```python
from build123d import *

# Parameters (mm, degrees)
SKETCH1_W           = 80
SKETCH1_H           = 40
BOSS_EXTRUDE1_DEPTH = 3
SKETCH2_W           = 80
SKETCH2_H           = 3
BOSS_EXTRUDE2_DEPTH = 12
SKETCH3_R           = 2
CUT_EXTRUDE1_DEPTH  = 12


with BuildPart() as part:
    # Sketch1 → Boss-Extrude1 (new body)
    with BuildSketch(Plane.XY):
        Rectangle(SKETCH1_W, SKETCH1_H)
    extrude(amount=BOSS_EXTRUDE1_DEPTH)

    # Sketch2 → Boss-Extrude2 (add)
    with BuildSketch(Plane.XY.offset(3)):
        with Locations((0, 18.5)):
            Rectangle(SKETCH2_W, SKETCH2_H)
    extrude(amount=BOSS_EXTRUDE2_DEPTH)

    # Sketch3 → Cut-Extrude1 (cut)
    with BuildSketch(Plane(origin=(0, 20, 0), x_dir=(1, 0, 0), z_dir=(0, 1, 0))):
        with Locations(Location((15, -8.5, 0), (0, 0, 270))):
            Circle(SKETCH3_R)
        with Locations(Location((-20, -8.5, 0), (0, 0, 270))):
            Circle(SKETCH3_R)
    extrude(amount=-CUT_EXTRUDE1_DEPTH, mode=Mode.SUBTRACT)


solid = part.part
```
Could you check a few things on this model? Use its own coordinates, in mm. A direction names the side the tool comes from. Give positions to 0.01 mm unless a question says otherwise; leave off trailing zeros. Loops run counter-clockwise (first coordinate to the right, second up) from the corner with the lowest first, then second, coordinate; pieces in that order, holes last. Notation, with made-up numbers: (86, 88) - (96, 88) arc R14 ccw to (96, 110) - close; hole circle Ø9 at (0, 88.5). An arc over 180 degrees is marked (long way). Answer in a Markdown table with one row per item. Add a question column.
Q1. For pin 1 (8 mm diameter, centred on y = -4, z = 4, fed in from -X); pin 2 (3 mm diameter, centred on x = -6, z = 9.5, fed in from -Y); pin 3 (3 mm diameter, centred on x = -20, z = 8.5, fed in from +Y); pin 4 (11 mm diameter, centred on x = 2.5, y = 7, fed in from +Z), each with a flat end and sliding along its axis, tell me the tip position at first contact or that it passes through.
Q2. Please list where these lines run through material, in increasing order: L1, parallel to X at y = 19.2, z = 8.5; L2, parallel to Y at x = -24.5, z = 13.5; L3, parallel to Z at x = 12, y = -10. Write a range as from..to.
Q3. If we section it at B-B (z = 8.5): List the corners of the cut face in (x, y) for me, plus the area to 3 significant figures.
Q4. If we section it at C-C (x = -2): List the corners of the cut face in (y, z) for me, plus the area to 3 significant figures.
Q5. If we section it at A-A (x = -20): List the corners of the cut face in (y, z) for me.
Q6. We'd pull the mould along Z, two halves only. Please class faces 1 (the face through (-1, -1, 3)), 2 (the face through (-18.017, 18.521, 8.24)), 3 (the face through (-40, 4, 2)): +Z half, -Z half, draft (parallel to the pull), parting line (faces both ways), or undercut.
Q7. If we section it at D-D (y = -2.5): List the corners of the cut face in (x, z) for me.
Q8. Which directions (+Z, -Z, +X, -X, +Y, -Y) give clear straight access to the entire face, cutting with the end or side of a thin tool? Please do faces 4 (the face through (-1, 17, 9)), 5 (the face through (-1, 0, 0)).
The answers:
| question | item | result |
|---|---|---|
| 1 | pin 1 | stops at x = -40 |
| 1 | pin 2 | stops at y = 17 |
| 1 | pin 3 | passes through |
| 1 | pin 4 | stops at z = 3 |
| 2 | L1 | x = -40..-22, -18..13, 17..40 |
| 2 | L2 | y = 17..20 |
| 2 | L3 | z = 0..3 |
| 3 | outline | (-40, 17) - (-22, 17) - (-22, 20) - (-40, 20) - close; (-18, 17) - (13, 17) - (13, 20) - (-18, 20) - close; (17, 17) - (40, 17) - (40, 20) - (17, 20) - close |
| 3 | area | 216 mm^2 |
| 4 | outline | (-20, 0) - (20, 0) - (20, 15) - (17, 15) - (17, 3) - (-20, 3) - close |
| 4 | area | 156 mm^2 |
| 5 | outline | (-20, 0) - (20, 0) - (20, 6.5) - (17, 6.5) - (17, 3) - (-20, 3) - close; (17, 10.5) - (20, 10.5) - (20, 15) - (17, 15) - close |
| 6 | face 1 | +Z half |
| 6 | face 2 | undercut |
| 6 | face 3 | draft |
| 7 | outline | (-40, 0) - (40, 0) - (40, 3) - (-40, 3) - close |
| 8 | face 4 | +Z, +X, -X, -Y |
| 8 | face 5 | -Z, +X, -X, +Y, -Y |
